Read the model definition and answer for the solid it produces. Units are mm, in the model's axes. Face numbers are marked on the shaded views. A direction names the side the tool comes from. Coordinates: 2 decimals unless noted, no trailing zeros. Write each loop counter-clockwise with the first axis right and the second up, starting at its lowest first coordinate (ties: lowest second). Pieces come first, ordered by that corner, then holes. Notation, with made-up numbers: (-20.5, 80) -> (15.5, 80) arc R24 cw to (15.5, 99) -> close; hole circle Ø8 at (-37, 27.25). An arc over 180 degrees is marked (long way). Answer in a Markdown table with one row per item. Add a question column.
Item 1: Straight lines are drawn through the part: line 1 (Y direction, x = 4.5, z = -4.5); line 2 (X direction, y = 7, z = -13.75). For each, find the intervals that lie inside material, in ascending order. Write a range as from..to.
Item 2: Section B-B on z = -11 is taken. Write down the section's boundary in (x, y).
Item 3: For a pull along Y with two mould halves and no side action, classify the marked faces 3, 4 and 5 as +Y half, -Y half, draft (parallel to the pull), parting line (faces both ways), or undercut.
Item 4: Given pin 1 Ø3 at (y, z) = (7.5, -11.5) entering from +X, flat-ended and moving along its own axis, determine where the tip first touches the part or whether it passes through.
Item 5: Section A-A on x = 7.75 is taken. Write down the section's boundary in (y, z).
Item 6: Section C-C on y = 6.25 is taken. Write down the section's boundary in (x, z).
Item 7: Which of the six approach directions +Z, -Z, +X, -X, +Y, -Y give full straight-line access (tool end or side, diameter ignored) to the marked faces 1 and 2?
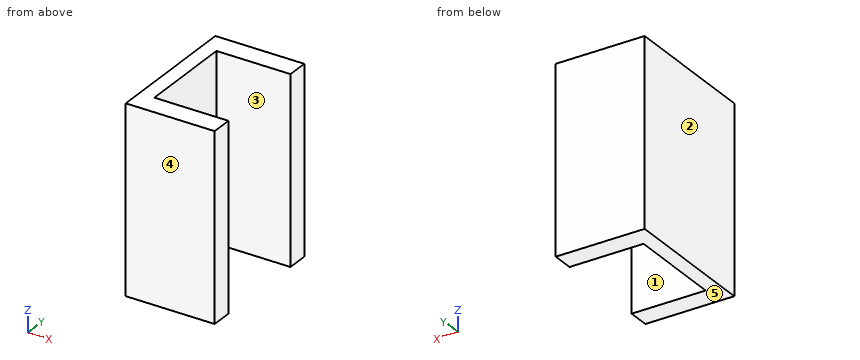
Autodesk Inventor part; units mm, degrees
ref_plane "YZ Plane" through (0, 0, 0) normal (1, 0, 0) x (0, 1, 0)
ref_plane "XZ Plane" through (0, 0, 0) normal (0, 1, 0) x (-1, 0, 0)
ref_plane "XY Plane" through (0, 0, 0) normal (0, 0, 1) x (1, 0, 0)
sketch "Sketch1" plane through (0, 0, 0) normal (1, 0, 0) x (0, 1, 0)
  line L0 (0, 0) -> (15, 0)
  line L1 (15, 0) -> (15, -20)
  line L2 (15, -20) -> (0, -20)
  line L3 (0, -20) -> (0, 0)
  dimension "d0" = 15
  dimension "d1" = 20
extrude "Extrusion1" add sketch "Sketch1" along normal blind 1.6
sketch "Sketch2" plane through (1.6, 0, 0) normal (1, 0, 0) x (0, 0, -1)
  line L0 (0, 15) -> (0, 0)
  line L1 (0, 0) -> (20, 0)
  line L2 (20, 0) -> (20, 15)
  line L3 (20, 15) -> (0, 15)
  line L4 (0, 15) -> (20, 15)
  line L5 (20, 15) -> (20, 12.7)
  line L6 (20, 12.7) -> (0, 12.7)
  line L7 (0, 12.7) -> (0, 15)
  line L8 (20, 0) -> (0, 0)
  line L9 (0, 0) -> (0, 2.3)
  line L10 (0, 2.3) -> (20, 2.3)
  line L11 (20, 2.3) -> (20, 0)
  dimension "d4" = 2.3
  dimension "d5" = 2.3
extrude "Extrusion2" add sketch "Sketch2" along normal blind 8 contours L3 L2 L6 L0 | L10 L2 L1 L0
equation "\"d5\" = d4"
properties part number "StepperDriverA4988"
Results below:
| question | item | result |
|---|---|---|
| 1 | line 1 | y = 0..2.3, 12.7..15 |
| 1 | line 2 | x = 0..1.6 |
| 2 | outline | (0, 0) -> (9.6, 0) -> (9.6, 2.3) -> (1.6, 2.3) -> (1.6, 12.7) -> (9.6, 12.7) -> (9.6, 15) -> (0, 15) -> close |
| 3 | face 3 | undercut |
| 3 | face 4 | -Y half |
| 3 | face 5 | draft |
| 4 | pin 1 | stops at x = 1.6 |
| 5 | outline | (0, -20) -> (2.3, -20) -> (2.3, 0) -> (0, 0) -> close; (12.7, -20) -> (15, -20) -> (15, 0) -> (12.7, 0) -> close |
| 6 | outline | (0, -20) -> (1.6, -20) -> (1.6, 0) -> (0, 0) -> close |
| 7 | face 1 | +Z, -Z, +X |
| 7 | face 2 | +Z, -Z, -X, +Y, -Y |
